The figure shows three views and two pictorial views of one solid part (mm, origin at its lowest corner). Answer the questions. A direction names the side the tool comes from. Coordinates: 2 decimals unless noted, no trailing zeros. Order: outer loops, then holes, each group sorted by start corner. A loop starts at its lowest first (then second) coordinate and runs counter-clockwise, first axis right, second up.
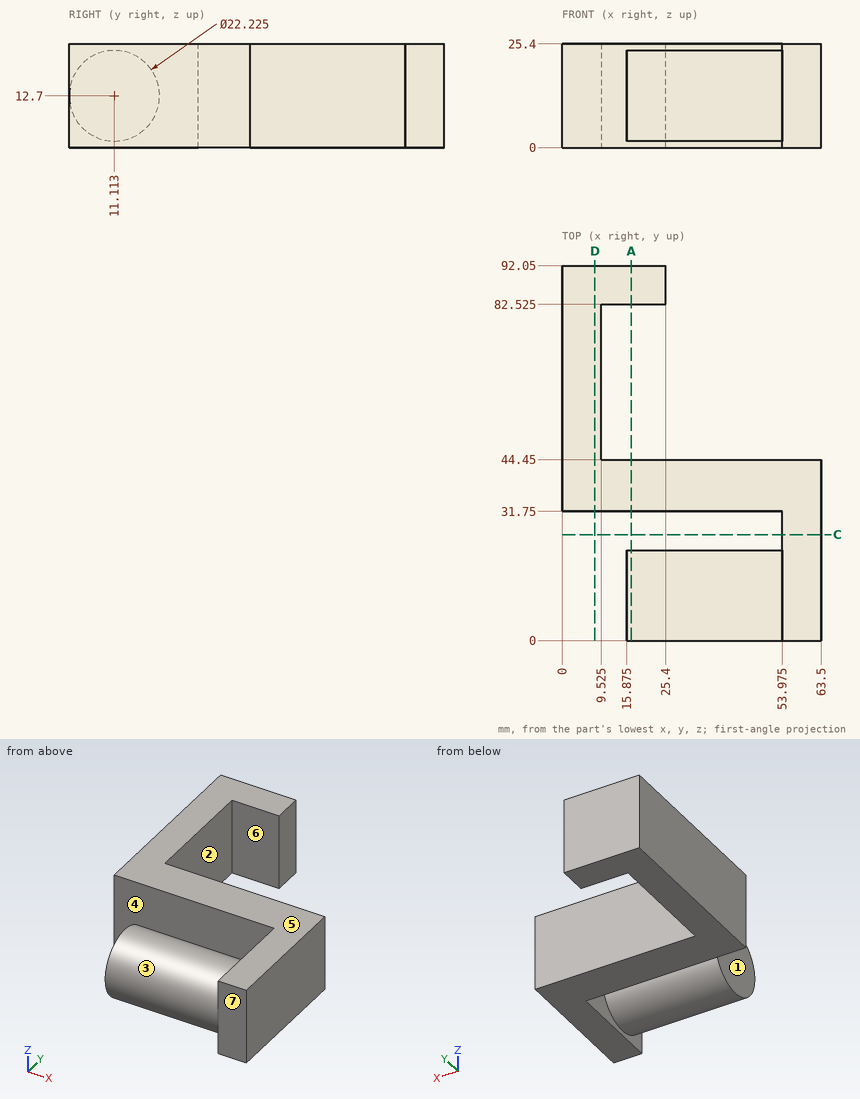
Q1. Determine the mould class of the marked faces 5, 6 and 7 for opening direction Y: +Y half, -Y half, draft (parallel to the pull), parting line (faces both ways), or undercut.
Q2. The part is cut by section D-D, the plane x = 8. Determine the outline of the cut face in (y, z), then the cut area to 3 significant figures.
Q3. Each of these flat-tipped pins is pushed along its axis until it touches: P1, Ø1, axis at y = 57.5, z = 3, coming from the +X side (1 decimal); P2, Ø1, axis at x = 52, z = 22, coming from the -Y side (1 decimal); P3, Ø2, axis at x = 10, z = 22, coming from the -Y side. Where does it stop, or does it pass through?
Q4. Which of the six approach directions +Z, -Z, +X, -X, +Y, -Y give full straight-line access (tool end or side, diameter ignored) to the marked faces 1, 2, 3 and 4?
Q5. Straight lines are drawn through the part: L1, parallel to X at y = 14, z = 11 (1 decimal); L2, parallel to X at y = 56, z = 8.75 (1 decimal); L3, parallel to Y at x = 5, z = 9.25. For each, find the intervals that lie inside material, in ascending order.
Q6. The part is cut by section A-A, the plane x = 17. State how many separate pieces and enclosed holes the cut face has.
Q7. The part is cut by section C-C, the plane y = 26. Determine the outline of the cut face in (x, z) (1 decimal), then the cut area to 3 significant figures.
Computed values:
1. face 5: draft
1. face 6: undercut
1. face 7: -Y half
2. outline: (31.75, 0) - (92.05, 0) - (92.05, 25.4) - (31.75, 25.4) - close
2. area: 1,530 mm2
3. P1: stops at x = 9.5
3. P2: stops at y = 4.3
3. P3: stops at y = 31.75
4. face 1: +Z, -Z, -X, -Y
4. face 2: +Z, -Z, +X
4. face 3: -X
4. face 4: +Z, -Z, -X
5. L1: x = 15.9 to 63.5
5. L2: x = 0 to 9.5
5. L3: y = 31.75 to 92.05
6. separate pieces: 3
6. enclosed holes: 0
7. outline: (54, 0) - (63.5, 0) - (63.5, 25.4) - (54, 25.4) - close
7. area: 242 mm2
